```python
from build123d import *

# Parameters (mm, degrees)
SKETCH_W     = 14
SKETCH_H     = 14
SKETCH_W_2   = 3
SKETCH_H_2   = 7
PAD_DEPTH    = 2
SKETCH006_R  = 4
PAD001_DEPTH = 20


with BuildPart() as part:
    # Sketch → Pad (new body)
    with BuildSketch(Plane.XY):
        Polygon((64, 0), (64, 84), (52, 84), (52, 74), (12, 74), (12, 84), (0, 84), (0, 0), (12, 0), (12, 10), (52, 10), (52, 0), align=None)
        with Locations((19, 55)):
            Rectangle(SKETCH_W, SKETCH_H, mode=Mode.SUBTRACT)
        with Locations((45, 55)):
            Rectangle(SKETCH_W, SKETCH_H, mode=Mode.SUBTRACT)
        with Locations((19, 29)):
            Rectangle(SKETCH_W, SKETCH_H, mode=Mode.SUBTRACT)
        with Locations((45, 29)):
            Rectangle(SKETCH_W, SKETCH_H, mode=Mode.SUBTRACT)
        with Locations((8.5, 5.5)):
            Rectangle(SKETCH_W_2, SKETCH_H_2, mode=Mode.SUBTRACT)
        with Locations((55.5, 5.5)):
            Rectangle(SKETCH_W_2, SKETCH_H_2, mode=Mode.SUBTRACT)
        with Locations((55.5, 78.5)):
            Rectangle(SKETCH_W_2, SKETCH_H_2, mode=Mode.SUBTRACT)
        with Locations((8.5, 78.5)):
            Rectangle(SKETCH_W_2, SKETCH_H_2, mode=Mode.SUBTRACT)
    extrude(amount=PAD_DEPTH)

    # Sketch006 → Pad001 (join)
    with BuildSketch(Plane.XY.offset(2)):
        with Locations((32, 42)):
            Circle(SKETCH006_R)
    extrude(amount=PAD001_DEPTH)


solid = part.part
```
Read the model definition and answer for the solid it produces. Units are mm, in the model's axes. A direction names the side the tool comes from. Give positions to 0.01 mm unless a question says otherwise; leave off trailing zeros. Write each loop counter-clockwise with the first axis right and the second up, starting at its lowest first coordinate (ties: lowest second). Pieces come first, ordered by that corner, then holes. Notation, with made-up numbers: (35.5, 15.25) - (86.5, 15.25) arc R21 cw to (86.5, 19.25) - close; hole circle Ø4 at (-32.5, 56.25). An arc over 180 degrees is marked (long way). Write item = value, one per line. Start each with the question number.
Item 1: Each of these flat-tipped pins is pushed along its axis until it touches: P1, Ø8, axis at x = 17, y = 29, coming from the -Z side; P2, Ø1.6, axis at x = 47, z = 1.5, coming from the -Y side; P3, Ø10, axis at x = 50, y = 70.5, coming from the +Z side; P4, Ø1, axis at x = 39, z = 1, coming from the +Y side. Where does it stop, or does it pass through?
Item 2: A tool of negligible diameter and unlimited length cuts with its end or side. For faces 1 (the flat face through (32, 43, 0)), 2 (the flat face through (52, 5, 1)), 3 (the flat face through (6, 0, 1)), 4 (the flat face through (19, 62, 1)), 5 (the flat face through (32, 74, 1)), from which of +Z, -Z, +X, -X, +Y, -Y can it reach the whole face along a straight path? Write none if from no direction.
Item 3: Find section B-B (y = 78.5). Give the vertices of the cut face in (x, z), then the cut area to 3 significant figures.
Item 4: Find section D-D (y = 42). Give the vertices of the cut face in (x, z).
Item 5: Find the intervals of material crossed by probe 1 along Z at (x, y) = (34, 35.5); probe 2 along X at (y, z) = (43, 5); probe 3 along Y at (x, z) = (30.5, 5.75), in increasing order. Write a range as [from, to].
Item 6: Find section A-A (x = 16). Give the vertices of the cut face in (y, z).
Item 7: Find section C-C (x = 32). Give the vertices of the cut face in (y, z), then the cut area to 3 significant figures.
Item 8: The mould has two halves that part along Y. Classify faces 6 (the flat face through (32, 42, 22)), 7 (the flat face through (7, 78, 1)), 8 (the flat face through (6, 84, 1)), 9 (the flat face through (7, 5, 1)): +Y half, -Y half, draft (parallel to the pull), parting line (faces both ways), or undercut.
Response:
q1.P1 = through
q1.P2 = 10
q1.P3 = 2
q1.P4 = 74
q2.face_1 = -Z, +X, -X, +Y, -Y
q2.face_2 = +Z, -Z, -Y
q2.face_3 = +Z, -Z, +X, -X, -Y
q2.face_4 = +Z, -Z
q2.face_5 = +Z, -Z, +Y
q3.outline = (0, 0) - (7, 0) - (7, 2) - (0, 2) - close; (10, 0) - (12, 0) - (12, 2) - (10, 2) - close; (52, 0) - (54, 0) - (54, 2) - (52, 2) - close; (57, 0) - (64, 0) - (64, 2) - (57, 2) - close
q3.area = 36.0 mm²
q4.outline = (0, 0) - (64, 0) - (64, 2) - (36, 2) - (36, 22) - (28, 22) - (28, 2) - (0, 2) - close
q5.probe_1 = [0, 2]
q5.probe_2 = [28.13, 35.87]
q5.probe_3 = [38.29, 45.71]
q6.outline = (10, 0) - (22, 0) - (22, 2) - (10, 2) - close; (36, 0) - (48, 0) - (48, 2) - (36, 2) - close; (62, 0) - (74, 0) - (74, 2) - (62, 2) - close
q7.outline = (10, 0) - (74, 0) - (74, 2) - (46, 2) - (46, 22) - (38, 22) - (38, 2) - (10, 2) - close
q7.area = 288 mm²
q8.face_6 = draft
q8.face_7 = undercut
q8.face_8 = +Y half
q8.face_9 = undercut
